Geometry check sheet. Reference: the model listing, model coordinates, mm. A direction names the side the tool comes from. Round coordinates to 2 decimals unless told otherwise and drop trailing zeros. Loops run counter-clockwise (first coordinate to the right, second up) from the corner with the lowest first, then second, coordinate; pieces in that order, holes last.
```python
from build123d import *

# Parameters (mm, degrees)
EXTRUDE_1_DEPTH          = 5
EXTRUDE_1_DEPTH_BACK     = 5
EXTRUDE_2_DEPTH          = 2
EXTRUDE_2_DEPTH_BACK     = 2
CUT_EXTRUDE_1_DEPTH      = 2
CUT_EXTRUDE_1_DEPTH_BACK = 2
SKETCH_5_R               = 4
SKETCH_5_R_2             = 2
EXTRUDE_3_DEPTH          = 16
EXTRUDE_4_DEPTH          = 1
EXTRUDE_4_DEPTH_BACK     = 1
CUT_EXTRUDE_2_REACH      = 41.97
CUT_EXTRUDE_START        = -16
SKETCH_7_R               = 2.5
CUT_EXTRUDE_3_REACH      = 25.97
SKETCH_8_R               = 2
FILLET_3_R               = 0.2
FILLET_5_R               = 0.2
FILLET_7_R               = 0.2
FILLET_8_R               = 0.1


with BuildPart() as part:
    # 草图1 → 凸台-拉伸1 (new, two sides: drawn at the far end of the back side and taken through both)
    with BuildSketch(Plane.XY.offset(-EXTRUDE_1_DEPTH_BACK)):
        Polygon((0, 0), (5.5, 0), (5.5, 2), (-11.647346039, 2), (-12, 0), align=None)
    extrude(amount=EXTRUDE_1_DEPTH + EXTRUDE_1_DEPTH_BACK)

    # 草图2 → 凸台-拉伸2 (add, two sides: drawn at the far end of the back side and taken through both)
    with BuildSketch(Plane.XY.offset(-EXTRUDE_2_DEPTH_BACK)):
        with BuildLine():
            Line((-1.5, 0), (1.5, 0))
            Line((1.5, 0), (1.5, -0.677124344))
            ThreePointArc((1.5, -0.677124344), (1.780042303, -1.088161527), (1.95, -1.555590279))
            Line((1.95, -1.555590279), (1.95, -2.5))
            Line((1.95, -2.5), (-1.95, -2.5))
            Line((-1.95, -2.5), (-1.95, -1.555590279))
            ThreePointArc((-1.95, -1.555590279), (-1.780042303, -1.088161527), (-1.5, -0.677124344))
            Line((-1.5, -0.677124344), (-1.5, 0))
        make_face()
    extrude(amount=EXTRUDE_2_DEPTH + EXTRUDE_2_DEPTH_BACK)

    # 草图3 → 切除-拉伸1 (cut, two sides: drawn at the far end of the back side and taken through both)
    with BuildSketch(Plane(origin=(0, 0, 0), x_dir=(0, 0, -1), z_dir=(1, 0, 0)).offset(-CUT_EXTRUDE_1_DEPTH_BACK)):
        with BuildLine():
            Line((1.5, 0), (1.5, -0.677124344))
            ThreePointArc((1.5, -0.677124344), (1.780042303, -1.088161527), (1.95, -1.555590279))
            Line((1.95, -1.555590279), (1.95, -2.5))
            Line((1.95, -2.5), (2, -2.5))
            Line((2, -2.5), (2, 0))
            Line((2, 0), (1.5, 0))
        make_face()
        with BuildLine():
            Line((-2, 0), (-1.5, 0))
            Line((-1.5, 0), (-1.5, -0.677124344))
            ThreePointArc((-1.5, -0.677124344), (-1.780042303, -1.088161527), (-1.95, -1.555590279))
            Line((-1.95, -1.555590279), (-1.95, -2.5))
            Line((-1.95, -2.5), (-2, -2.5))
            Line((-2, -2.5), (-2, 0))
        make_face()
    extrude(amount=CUT_EXTRUDE_1_DEPTH + CUT_EXTRUDE_1_DEPTH_BACK, mode=Mode.SUBTRACT)

    # 草图5 → 凸台-拉伸3 (add)
    with BuildSketch(Plane(origin=(-11.647346039, 2, 5), x_dir=(-0.9848077530122089, 0.17364817766692556, 0), z_dir=(-0.17364817766692556, -0.984807753012209, 0))):
        with Locations(Location((-4.4, 5, 0), (0, 0, 180))):
            Circle(SKETCH_5_R)
        with Locations(Location((-4.4, 5, 0), (0, 0, 180))):
            Circle(SKETCH_5_R_2, mode=Mode.SUBTRACT)
    extrude(amount=-EXTRUDE_3_DEPTH)

    # 草图6 → 凸台-拉伸4 (add, two sides: drawn at the far end of the back side and taken through both)
    with BuildSketch(Plane.XY.offset(-EXTRUDE_4_DEPTH_BACK)):
        Polygon((5.5, 2), (-0.596590071, 16.298279356), (-2.0738017, 16.558751622), (-4.640902417, 2), align=None)
    extrude(amount=EXTRUDE_4_DEPTH + EXTRUDE_4_DEPTH_BACK)

    # 切除-拉伸2: up to this plane
    cut_extrude_2_end = Plane(origin=(0, 0, -5), z_dir=(0, -1, 0))
    # 草图7 → 切除-拉伸2 (cut, up to the surface)
    with BuildSketch(Plane(origin=(2.769180529, 15.704803188, 0), x_dir=(0.9848077530122089, -0.17364817766692558, 0), z_dir=(0.17364817766692558, 0.984807753012209, 0)).offset(CUT_EXTRUDE_START), mode=Mode.PRIVATE) as cut_extrude_2_sk1:
        with Locations(Location((-7.417693036, 0, 0), (0, 0, 180))):
            Circle(SKETCH_7_R)
    cut_extrude_2_tool1 = split(extrude(cut_extrude_2_sk1.sketch, amount=-CUT_EXTRUDE_2_REACH, mode=Mode.PRIVATE), bisect_by=cut_extrude_2_end, keep=Keep.BOTH, mode=Mode.PRIVATE)
    add(cut_extrude_2_tool1.solids().sort_by_distance((-7.314192, 1.235948, 0))[0], mode=Mode.SUBTRACT)

    # 草图8 → 切除-拉伸3 (cut, up to next)
    with BuildSketch(Plane(origin=(2.769180529, 15.704803188, 0), x_dir=(0.9848077530122089, -0.17364817766692558, 0), z_dir=(0.17364817766692558, 0.984807753012209, 0)), mode=Mode.PRIVATE) as cut_extrude_3_sk1:
        with Locations((-7.417693036, 0)):
            Circle(SKETCH_8_R)
    cut_extrude_3_tool1 = extrude(cut_extrude_3_sk1.sketch, amount=-CUT_EXTRUDE_3_REACH, mode=Mode.PRIVATE) & part.part
    add(cut_extrude_3_tool1.solids().sort_by_distance((-4.535821, 16.992872, 0))[0], mode=Mode.SUBTRACT)

    # 圆角3
    fillet_3_edges = [part.edges().sort_by_distance(p)[0] for p in [
        (5.5, 1, -5),
        (-3.073673019, 2, -5),
        (-3.25, 0, 5),
        (5.5, 1, 5),
        (-11.823673019, 1, -5),
        (-3.073673019, 2, 5),
        (-11.823673019, 1, 5),
        (-3.25, 0, -5),
        (-12, 0, 0),
        (-11.647346039, 2, 0),
    ]]
    fillet(fillet_3_edges, radius=FILLET_3_R)

    # 圆角5
    # the kernel refuses this fillet: 0.2 mm, written as the material it takes off along each edge
    with BuildSketch(Plane(origin=(5.3, 0.2, 4.8), x_dir=(1, 0, 0), z_dir=(0, -1, 0))) as fillet_5_piece_1_section:
        Polygon((0, 0), (FILLET_5_R, 0), (FILLET_5_R, FILLET_5_R), (0, FILLET_5_R), align=None)
    fillet_5_piece_1 = extrude(amount=FILLET_5_R, mode=Mode.PRIVATE)
    fillet_5_piece_1 = fillet_5_piece_1 - Plane(origin=(5.3, 0.2, 4.8), x_dir=(-0.7071067811865475, 0, -0.7071067811865475), z_dir=(0, -1, 0)) * Sphere(FILLET_5_R, mode=Mode.PRIVATE)
    add(fillet_5_piece_1, mode=Mode.SUBTRACT)
    with BuildSketch(Plane(origin=(5.3, 0.2, -4.8), x_dir=(1, 0, 0), z_dir=(0, -1, 0))) as fillet_5_piece_2_section:
        Polygon((0, 0), (FILLET_5_R, 0), (FILLET_5_R, -FILLET_5_R), (0, -FILLET_5_R), align=None)
    fillet_5_piece_2 = extrude(amount=FILLET_5_R, mode=Mode.PRIVATE)
    fillet_5_piece_2 = fillet_5_piece_2 - Plane(origin=(5.3, 0.2, -4.8), x_dir=(-0.7071067811865475, 0, 0.7071067811865475), z_dir=(0, -1, 0)) * Sphere(FILLET_5_R, mode=Mode.PRIVATE)
    add(fillet_5_piece_2, mode=Mode.SUBTRACT)
    with BuildSketch(Plane(origin=(5.5, 0, -4.8), x_dir=(-1, 0, 0), z_dir=(0, 0, 1))) as fillet_5_piece_3:
        with BuildLine():
            CenterArc((FILLET_5_R, -FILLET_5_R), FILLET_5_R, 90, 90)
            Line((0, -FILLET_5_R), (0, 0))
            Line((0, 0), (FILLET_5_R, 0))
        make_face()
    extrude(amount=9.6, mode=Mode.SUBTRACT)

    # 圆角7
    # the kernel refuses this fillet: 0.2 mm, written as the material it takes off along each edge
    with BuildSketch(Plane(origin=(-0.596590071, 16.298279356, -1.270954164), x_dir=(0.39222047204702226, -0.9198712417002779, 0), z_dir=(0, 0, 1))) as fillet_7_piece_1:
        with BuildLine():
            CenterArc((FILLET_7_R * 0.541908328714, -FILLET_7_R), FILLET_7_R, 90, 56.907265605)
            Line((-FILLET_7_R * 0.295879631671, -FILLET_7_R * 0.454004273429), (0, 0))
            Line((0, 0), (FILLET_7_R * 0.541908328714, 0))
        make_face()
    extrude(amount=2.541908329, mode=Mode.SUBTRACT)
    with BuildSketch(Plane(origin=(5.696110236, 1.540064379, -1), x_dir=(0, 0, 1), z_dir=(-0.39222047204701954, 0.9198712417002791, 0))) as fillet_7_piece_2_section:
        with BuildLine():
            CenterArc((FILLET_7_R, -FILLET_7_R), FILLET_7_R, 90, 90)
            Line((0, -FILLET_7_R), (0, 0))
            Line((0, 0), (FILLET_7_R, 0))
        make_face()
    fillet_7_piece_2 = extrude(amount=16.543783421, mode=Mode.PRIVATE)
    fillet_7_piece_2 = split(fillet_7_piece_2, bisect_by=Plane(origin=(2.402045939, 2, -0.955327029), z_dir=(0, 1, 0)), keep=Keep.TOP, mode=Mode.PRIVATE)
    fillet_7_piece_2 = fillet_7_piece_2 - Plane(origin=(-5.66753398, 10.574609288, 0), x_dir=(0.984807753012209, -0.17364817766692556, 0), z_dir=(-0.17364817766692556, -0.984807753012209, 0)) * Cylinder(4, 34, mode=Mode.PRIVATE)
    add(fillet_7_piece_2, mode=Mode.SUBTRACT)
    with BuildSketch(Plane(origin=(5.696110236, 1.540064379, 1), x_dir=(0, 0, -1), z_dir=(-0.39222047204701954, 0.9198712417002791, 0))) as fillet_7_piece_3_section:
        with BuildLine():
            CenterArc((FILLET_7_R, FILLET_7_R), FILLET_7_R, 180, 90)
            Line((0, FILLET_7_R), (0, 0))
            Line((0, 0), (FILLET_7_R, 0))
        make_face()
    fillet_7_piece_3 = extrude(amount=16.543783421, mode=Mode.PRIVATE)
    fillet_7_piece_3 = split(fillet_7_piece_3, bisect_by=Plane(origin=(2.402045936, 2, 0.955327029), z_dir=(0, 1, 0)), keep=Keep.TOP, mode=Mode.PRIVATE)
    fillet_7_piece_3 = fillet_7_piece_3 - Plane(origin=(-5.667533979, 10.574609294, 0), x_dir=(0.984807753012209, -0.17364817766692556, 0), z_dir=(-0.17364817766692556, -0.984807753012209, 0)) * Cylinder(4, 34, mode=Mode.PRIVATE)
    add(fillet_7_piece_3, mode=Mode.SUBTRACT)

    # 圆角8
    fillet_8_edges = [part.edges().sort_by_distance(p)[0] for p in [
        (0, -2.5, 1.95),
        (1.95, -2.5, 0),
        (-1.95, -2.5, 0),
        (0, -2.5, -1.95),
    ]]
    fillet(fillet_8_edges, radius=FILLET_8_R)


solid = part.part
```
1) Access from +Z, -Z, +X, -X, +Y, -Y to the whole of each face (thin tool, end or side, straight path). Record for faces 5 (the face through (1.95, -2, 0)), 6 (the face through (-0.027, -1.082, 1.777)), 7 (the face through (0, -2, -1.95)), 8 (the face through (-1.95, -2, 0)), 9 (the face through (1.777, -1.082, -0.027)).
Report:
face 5: +Z, -Z, +X, -Y
face 6: +Z, +X, -X
face 7: -Z, +X, -X, -Y
face 8: +Z, -Z, -X, -Y
face 9: +Z, -Z, +X
2) Mould release check, pull along Y, two halves, no side actions. Record for faces 1 (the face through (1, 6, 1)), 2 (the face through (0, -2.5, 0)), 3 (the face through (5.5, 1, 0)), 4 (the face through (2.43, 9.06, -0.94)): +Y half, -Y half, draft (parallel to the pull), parting line (faces both ways), or undercut.
Report:
face 1: undercut
face 2: -Y half
face 3: draft
face 4: +Y half
3) Sectioned sample at A-A, the plane z = -3.25. Record the cut outline in (x, y), then the cut area to 3 significant figures.
Report:
outline: (-11.96, 0.23) arc R0.2 ccw to (-11.76, 0) - (5.3, 0) arc R0.2 ccw to (5.5, 0.2) - (5.5, 2) - (-4.81, 2) - (-2.24, 16.59) - (-6.83, 17.4) - (-9.55, 2) - (-11.48, 2) arc R0.2 ccw to (-11.68, 1.83) - close
area: 106 mm2
4) Gauge pin test, flat ends, axial feed: pin 1 (7 mm diameter, centred on x = -0.5, y = 8.5, fed in from +Z); pin 2 (0.7 mm diameter, centred on x = 0, y = -0.5, fed in from -Z); pin 3 (0.7 mm diameter, centred on y = -2, z = -1, fed in from -X); pin 4 (5 mm diameter, centred on y = -0.5, z = 0, fed in from +X). Record the tip position at first contact, or that the pin passes through.
Report:
pin 1: stops at z = 3.49
pin 2: stops at z = -1.64
pin 3: stops at x = -1.95
pin 4: stops at x = 5.5
5) Scan lines: line 1 along Y through (x, z) = (4.25, 2); line 2 along X through (y, z) = (10, 1.5); line 3 along Z through (x, y) = (-4, 15). Record each from-to range of solid material in increasing order.
Report:
line 1: y = 0 to 2
line 2: x = -9.53 to -7.11, -4.43 to -2
line 3: z = -3.9 to -1.8, 1.8 to 3.9
